Design review of the part built by this model. Coordinates are the model's own, in mm. A direction names the side the tool comes from. Give positions to 0.01 mm unless a question says otherwise; leave off trailing zeros. Order: outer loops, then holes, each group sorted by start corner. A loop starts at its lowest first (then second) coordinate and runs counter-clockwise, first axis right, second up.
```python
from build123d import *

# Parameters (mm, degrees)
BOSS_EXTRUDE1_DEPTH = 0.5
BOSS_EXTRUDE2_START = -3.85
BOSS_EXTRUDE2_DEPTH = 3.85
SKETCH2_R           = 1.15
CUT_EXTRUDE1_DEPTH  = 10
CUT_EXTRUDE2_START  = 3.85
CUT_EXTRUDE2_DEPTH  = 0.6


with BuildPart() as part:
    # Sketch1 → Boss-Extrude1 (new body)
    with BuildSketch(Plane(origin=(0, 0, 0), x_dir=(1, 0, 0), z_dir=(0, 1, 0))):
        with BuildLine():
            Line((-8, -2), (-7.480220773, 0.445369002))
            ThreePointArc((-7.480220773, 0.445369002), (-3.928611493, 2.234065485), (0, 2.85))
            ThreePointArc((0, 2.85), (2.760304316, -0.709380069), (-1.374108678, -2.4968631))
            ThreePointArc((-1.374108678, -2.4968631), (-4.633030541, -1.528000078), (-8, -2))
        make_face()
    extrude(amount=BOSS_EXTRUDE1_DEPTH)

    # Sketch1<3> → Boss-Extrude2 (add)
    with BuildSketch(Plane(origin=(0, 0, 0), x_dir=(1, 0, 0), z_dir=(0, 1, 0)).offset(BOSS_EXTRUDE2_START)):
        with BuildLine():
            Line((-8, -2), (-7.480220773, 0.445369002))
            ThreePointArc((-7.480220773, 0.445369002), (-3.928611493, 2.234065485), (0, 2.85))
            ThreePointArc((0, 2.85), (2.760304316, -0.709380069), (-1.374108678, -2.4968631))
            ThreePointArc((-1.374108678, -2.4968631), (-4.633030541, -1.528000078), (-8, -2))
        make_face()
        with BuildLine():
            Line((-6.516291445, 0.083732705), (-1.181900943, 1.423239319))
            ThreePointArc((-1.181900943, 1.423239319), (1.501730026, -1.080419793), (-1.725107949, 0.668208473))
            Line((-1.725107949, 0.668208473), (-6.370163451, -0.498200805))
            Line((-6.370163451, -0.498200805), (-6.516291445, 0.083732705))
        make_face(mode=Mode.SUBTRACT)
    extrude(amount=BOSS_EXTRUDE2_DEPTH)

    # Sketch2 → Cut-Extrude1 (cut)
    with BuildSketch(Plane.XZ):
        with Locations(Location((0, 0, 0), (0, 0, 270))):
            Circle(SKETCH2_R)
    extrude(amount=-CUT_EXTRUDE1_DEPTH, mode=Mode.SUBTRACT)

    # Sketch3 → Cut-Extrude2 (cut)
    with BuildSketch(Plane.XZ.offset(CUT_EXTRUDE2_START)):
        with BuildLine():
            Line((1.085530532, 0.832876632), (1.48692434, 2.431369163))
            ThreePointArc((1.48692434, 2.431369163), (1.944053318, 2.08402416), (2.322291558, 1.652108326))
            Line((2.322291558, 1.652108326), (1.794294987, -0.450561316))
            Line((1.794294987, -0.450561316), (1.085530532, 0.832876632))
        make_face()
    extrude(amount=-CUT_EXTRUDE2_DEPTH, mode=Mode.SUBTRACT)


solid = part.part
```
1. Machinability: for faces 5 (the face through (1.544, -1.952, 1.019)), 6 (the face through (-2, 0.5, 0)), which of the approach directions +Z, -Z, +X, -X, +Y, -Y give a long, thin tool a straight path to every point of the face, cutting with its end or side? Answer none if there is none.
Recorded:
face 5: -Y
face 6: +Z, -Z, +X, -X, +Y
2. Take a section at C-C (y = -0.95). State the section outline as (x, z) points.
Recorded:
outline: (-8, 2) - (-7.48, -0.45) arc R12.84 ccw to (0, -2.85) arc R2.85 ccw (long way) to (-1.37, 2.5) arc R8 cw to start; hole (-6.52, -0.08) - (-1.18, -1.42) arc R1.85 ccw (long way) to (-1.73, -0.67) - (-6.37, 0.5) - close
3. Take a section at B-B (x = 0.5). State the section outline as (y, z) points, then the cut area to 3 significant figures.
Recorded:
outline: (-3.85, -2.81) - (0.5, -2.81) - (0.5, -1.04) - (0, -1.04) - (0, -1.78) - (-3.85, -1.78) - close; (-3.85, 1.78) - (0, 1.78) - (0, 1.04) - (0.5, 1.04) - (0.5, 2.81) - (-3.85, 2.81) - close
area: 9.66 mm2
4. Draft analysis for pull direction X (two halves, no side actions). For faces 1 (the face through (-2, -3.85, 0)), 2 (the face through (-7.744, -1.705, 0.794)), 3 (the face through (2, -3.25, 1)), 4 (the face through (-3.886, -1.952, -0.744)), state which applies: pulls with the +X half, pulls with the -X half, needs draft (parallel to the pull), parting line crosses it, or undercut.
Recorded:
face 1: needs draft
face 2: pulls with the -X half
face 3: undercut
face 4: undercut
5. Take a section at D-D (x = -2.5). State the section outline as (y, z) points, then the cut area to 3 significant figures.
Recorded:
outline: (-3.85, -2.6) - (0.5, -2.6) - (0.5, 1.99) - (-3.85, 1.99) - (-3.85, -0.47) - (0, -0.47) - (0, -1.09) - (-3.85, -1.09) - close
area: 17.6 mm2
6. For line 1 along Z through (x, y) = (0, -2.9); line 2 along Z through (x, y) = (-5, -1.55); line 3 along Y through (x, z) = (-0.5, 1.15), list the stretches that pass through material, from the lowest coordinate up.
Recorded:
line 1: z = -2.85 to -1.85, 1.85 to 2.85
line 2: z = -1.84 to -0.46, 0.15 to 1.51
line 3: y = 0 to 0.5
7. Take a section at A-A (y = 0.25). State the section outline as (x, z) points, then the cut area to 3 significant figures.
Recorded:
outline: (-8, 2) - (-7.48, -0.45) arc R12.84 ccw to (0, -2.85) arc R2.85 ccw (long way) to (-1.37, 2.5) arc R8 cw to start; hole circle Ø2.3 at (0, 0)
area: 39.2 mm2
8. For pin 1 (1 mm diameter, centred on x = -6.5, y = -1, fed in from +Z), flat-tipped, find the tip position at first contact; note if it passes through.
Recorded:
pin 1: stops at z = 1.7
